CAD build for the part. Positions are in the model's coordinates, mm. Give positions to 0.01 mm unless a question says otherwise; leave off trailing zeros. Order: outer loops, then holes, each group sorted by start corner. A loop starts at its lowest first (then second) coordinate and runs counter-clockwise, first axis right, second up.
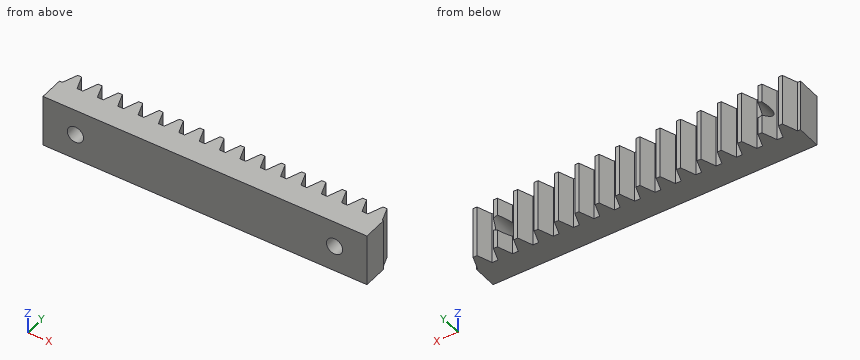
from build123d import *

# Parameters (mm, degrees)
BLANKSKE_W         = 50
BLANKSKE_H         = 6
BLANK_DEPTH        = 8
TOOTHCUTSIM_DEPTH  = 51.990195136
TEETHCUTS_COUNT    = 17
TEETHCUTS_PITCH    = 3.14159265
SKETCH1_R          = 1.25
CUT_EXTRUDE1_DEPTH = 10


with BuildPart() as part:
    # BlankSke → Blank (new body)
    with BuildSketch(Plane.XY):
        with Locations((25, 3)):
            Rectangle(BLANKSKE_W, BLANKSKE_H)
    extrude(amount=-BLANK_DEPTH)

    # TooCutSkeSim → ToothCutSim (cut, through all)
    with BuildSketch(Plane.XY):
        Polygon((0.44443537, 3.75), (-0.44443537, 3.75), (-1.272613241, 6.0254), (1.272613241, 6.0254), align=None)
    toothcutsim = extrude(amount=-TOOTHCUTSIM_DEPTH, mode=Mode.SUBTRACT)

    # TeethCuts: ToothCutSim ×17
    with Locations(*[(i * TEETHCUTS_PITCH, 0, 0) for i in range(1, TEETHCUTS_COUNT)]):
        add(toothcutsim, mode=Mode.SUBTRACT)

    # Sketch1 → Cut-Extrude1 (cut)
    with BuildSketch(Plane(origin=(0, 0, 0), x_dir=(-1, 0, 0), z_dir=(0, -1, 0))):
        with Locations(Location((-45, 4, 0), (0, 0, 90))):
            Circle(SKETCH1_R)
        with Locations(Location((-5, 4, 0), (0, 0, 90))):
            Circle(SKETCH1_R)
    extrude(amount=-CUT_EXTRUDE1_DEPTH, mode=Mode.SUBTRACT)


solid = part.part
1. Pin check, flat tips, straight feed: P1, Ø0.7, axis at x = 12.5, z = -3.5, coming from the +Y side; P2, Ø0.7, axis at x = 3.5, z = -4, coming from the +Y side. Stop position of each tip, or through.
2. Wall check: line 1 (Z direction, x = 45, y = 2.75); line 2 (Z direction, x = 4, y = 4); line 3 (Y direction, x = 16, z = -7.5). Give the ranges that are in metal, low to high.
3. Saw through at B-B on z = -4. State how many separate pieces and enclosed holes the cut face has, plus the area to 3 significant figures.
4. Saw through at A-A on y = 2. Give the cut face in (x, z), plus the area to 3 significant figures.
Reported:
1. P1: stops at y = 3.75
1. P2: stops at y = 4.26
2. line 1: z = -8 to -5.25, -2.75 to 0
2. line 2: z = -8 to -4.75, -3.25 to 0
2. line 3: y = 0 to 3.75
3. separate pieces: 3
3. enclosed holes: 0
3. area: 214 mm2
4. outline: (0, -8) - (50, -8) - (50, 0) - (0, 0) - close; hole circle Ø2.5 at (5, -4); hole circle Ø2.5 at (45, -4)
4. area: 390 mm2
